```python
from build123d import *

# Parameters (mm, degrees)
BOSS_EXTRUDE1_DEPTH = 11.5
BOSS_EXTRUDE2_DEPTH = 22
SKETCH3_R           = 2.5
CUT_EXTRUDE1_DEPTH  = 4
SKETCH4_R           = 4.5
CUT_EXTRUDE2_DEPTH  = 5
SKETCH5_R           = 2.75
CUT_EXTRUDE3_DEPTH  = 125.343311555
SKETCH6_R           = 2.5
CUT_EXTRUDE4_DEPTH  = 79.78509189
CUT_EXTRUDE5_DEPTH  = 8.2
CUT_EXTRUDE6_DEPTH  = 9
FILLET1_R           = 5.05
FILLET2_R           = 5


with BuildPart() as part:
    # Sketch1 → Boss-Extrude1 (new body)
    with BuildSketch(Plane(origin=(0, 0, 0), x_dir=(1, 0, 0), z_dir=(0, 1, 0))):
        with BuildLine():
            Line((66.174969976, -35), (93.674969976, -35))
            ThreePointArc((93.674969976, -35), (98.07852804, 19.509032202), (73.150467337, 68.183642675))
            Line((73.150467337, 68.183642675), (47.743780193, 57.659848285))
            ThreePointArc((47.743780193, 57.659848285), (73.422287359, 14.604600997), (66.174969976, -35))
        make_face()
    extrude(amount=BOSS_EXTRUDE1_DEPTH)

    # Sketch2 → Boss-Extrude2 (add)
    with BuildSketch(Plane.XZ.offset(-11.5)):
        with BuildLine():
            Line((80.428539711, 23.5), (86.877787725, 23.5))
            ThreePointArc((86.877787725, 23.5), (85.091202872, 29.317012019), (82.915619759, 35))
            Line((82.915619759, 35), (76.428539711, 35))
            Line((76.428539711, 35), (76.428539711, 27.5))
            ThreePointArc((76.428539711, 27.5), (77.600112586, 24.671572875), (80.428539711, 23.5))
        make_face()
        with BuildLine():
            Line((60.086969148, -54.654623051), (57.216843406, -61.583719545))
            Line((57.216843406, -61.583719545), (63.210123888, -64.066217604))
            ThreePointArc((63.210123888, -64.066217604), (67.394885944, -59.648380938), (71.271549248, -54.957859017))
            Line((71.271549248, -54.957859017), (65.313221008, -52.489838651))
            ThreePointArc((65.313221008, -52.489838651), (62.251753549, -52.489838651), (60.086969148, -54.654623051))
        make_face()
    extrude(amount=-BOSS_EXTRUDE2_DEPTH)

    # Sketch3 → Cut-Extrude1 (cut)
    with BuildSketch(Plane(origin=(0, 33.5, 0), x_dir=(1, 0, 0), z_dir=(0, 1, 0))):
        with Locations(Location((63.782487278, 56.185356781, 0), (0, 0, 270))):
            Circle(SKETCH3_R)
        with Locations(Location((80.428539711, -27.5, 0), (0, 0, 270))):
            Circle(SKETCH3_R)
    extrude(amount=-CUT_EXTRUDE1_DEPTH, mode=Mode.SUBTRACT)

    # Sketch4 → Cut-Extrude2 (cut)
    with BuildSketch(Plane.XZ):
        with Locations(Location((91.060743988, 27, 0), (0, 0, 270))):
            Circle(SKETCH4_R)
        with Locations(Location((73.796704912, -59.792185441, 0), (0, 0, 270))):
            Circle(SKETCH4_R)
    extrude(amount=-CUT_EXTRUDE2_DEPTH, mode=Mode.SUBTRACT)

    # Sketch5 → Cut-Extrude3 (cut, through all)
    with BuildSketch(Plane.XZ.offset(-5)):
        with Locations(Location((91.060743988, 27, 0), (0, 0, 270))):
            Circle(SKETCH5_R)
        with Locations(Location((73.796704912, -59.792185441, 0), (0, 0, 270))):
            Circle(SKETCH5_R)
    extrude(amount=-CUT_EXTRUDE3_DEPTH, mode=Mode.SUBTRACT)

    # Sketch6 → Cut-Extrude4 (cut, through all)
    with BuildSketch(Plane(origin=(56.959375084, 0, -11.329924142), x_dir=(0.19509032201612866, 0, 0.9807852804032304), z_dir=(-0.9807852804032304, 0, 0.19509032201612866))):
        with Locations((0, 7.5)):
            Circle(SKETCH6_R)
    extrude(amount=-CUT_EXTRUDE4_DEPTH, mode=Mode.SUBTRACT)

    # Sketch8 → Cut-Extrude5 (cut)
    with BuildSketch(Plane(origin=(98.07852804, 0, -19.509032202), x_dir=(-0.19509032201612866, 0, -0.9807852804032304), z_dir=(0.9807852804032304, 0, -0.19509032201612866))):
        with BuildLine():
            Line((-4.5, 7.5), (-4.5, 11.5))
            Line((-4.5, 11.5), (4.5, 11.5))
            Line((4.5, 11.5), (4.5, 7.5))
            ThreePointArc((4.5, 7.5), (0, 3), (-4.5, 7.5))
        make_face()
    extrude(amount=-CUT_EXTRUDE5_DEPTH, mode=Mode.SUBTRACT)

    # Sketch7 → Cut-Extrude6 (cut)
    with BuildSketch(Plane(origin=(0, 11.5, 0), x_dir=(1, 0, 0), z_dir=(0, 1, 0))):
        Polygon((69.47485004, 18.968342244), (71.445262293, 9.062410912), (79.291544536, 10.623133488), (77.321132284, 20.52906482), align=None)
    extrude(amount=-CUT_EXTRUDE6_DEPTH, mode=Mode.SUBTRACT)

    # Fillet1
    # the kernel refuses this fillet: 5.05 mm, written as the material it adds along each edge
    with BuildSketch(Plane(origin=(61.857828731, 2.5, -7.155351805), x_dir=(0, 1, 0), z_dir=(0.9807852804032302, 0, -0.1950903220161298))) as fillet1_piece_1_section:
        with BuildLine():
            CenterArc((FILLET1_R, -FILLET1_R), FILLET1_R, 90, 90)
            Line((0, -FILLET1_R), (0, 0))
            Line((0, 0), (FILLET1_R, 0))
        make_face()
    fillet1_piece_1 = extrude(amount=30.40026249, mode=Mode.PRIVATE)
    fillet1_piece_1 = fillet1_piece_1 - Plane(origin=(0, 3.649852304, 0), x_dir=(0.6377681563457176, 0, -0.7702283938880625), z_dir=(0, -1, 0)) * Cylinder(74.860715007, 82, mode=Mode.PRIVATE)
    add(fillet1_piece_1)
    with BuildSketch(Plane(origin=(89.703546449, 2.5, -22.992080135), x_dir=(0, 1, 0), z_dir=(-0.9807852804032304, 0, 0.19509032201612841))) as fillet1_piece_2_section:
        with BuildLine():
            CenterArc((FILLET1_R, -FILLET1_R), FILLET1_R, 90, 90)
            Line((0, -FILLET1_R), (0, 0))
            Line((0, 0), (FILLET1_R, 0))
        make_face()
    fillet1_piece_2 = extrude(amount=30.40026249, mode=Mode.PRIVATE)
    fillet1_piece_2 = fillet1_piece_2 - Plane(origin=(0, 3.643295327, 0), x_dir=(0.6377681563457176, 0, -0.7702283938880625), z_dir=(0, -1, 0)) * Cylinder(74.860715007, 82, mode=Mode.PRIVATE)
    add(fillet1_piece_2)

    # Fillet2
    fillet2_edges = [part.edges().sort_by_distance(p)[0] for p in [
        (66.174969976, 5.75, 35),
        (47.743780193, 5.75, -57.659848285),
    ]]
    fillet(fillet2_edges, radius=FILLET2_R)


solid = part.part
```
Could you check a few things on this model? Use its own coordinates, in mm. A direction names the side the tool comes from. Coordinates: 2 decimals unless noted, no trailing zeros. Loops run counter-clockwise (first coordinate to the right, second up) from the corner with the lowest first, then second, coordinate; pieces in that order, holes last.
1) Will these pins go through, and if not, where does the flat tip stop? pin 1 Ø4 at (x, z) = (80.43, 27.5) entering from +Y; pin 2 Ø2 at (y, z) = (11.5, -33.5) entering from -X; pin 3 Ø4.5 at (x, z) = (91.06, 27) entering from +Y; pin 4 Ø4 at (y, z) = (12, 10) entering from -X.
Reported:
pin 1: stops at y = 29.5
pin 2: stops at x = 66.44
pin 3: passes through
pin 4: stops at x = 73.9
2) Imagine slicing it at B-B (y = 31). List the corners of the cut face in (x, z) for me, and give its area (3 significant figures).
Reported:
outline: (57.22, -61.58) - (63.21, -64.07) arc R90 ccw to (71.27, -54.96) - (65.31, -52.49) arc R4 ccw to (60.09, -54.65) - close; (76.43, 27.5) arc R4 ccw to (80.43, 23.5) - (86.88, 23.5) arc R90 ccw to (82.92, 35) - (76.43, 35) - close; hole circle Ø5 at (63.78, -56.19); hole circle Ø5 at (80.43, 27.5)
area: 152 mm2
3) Thinking about a two-plate mould opening in Z: for faces 1 (the face through (69.83, 5.83, 32.74)), 2 (the face through (77.57, 22.35, 24.7)), 3 (the face through (85.119, 22.346, 29.236)), which applies, released by +Z, released by -Z, zero draft, split by the parting line, or undercut?
Reported:
face 1: undercut
face 2: released by -Z
face 3: released by +Z
4) Imagine slicing it at C-C (z = 2). List the corners of the cut face in (x, y) for me, and give its area (3 significant figures).
Reported:
outline: (74.83, 0) - (99.98, 0) - (99.98, 11.5) - (74.83, 11.5) - close
area: 289 mm2
5) Which directions (+Z, -Z, +X, -X, +Y, -Y) give clear straight access to the entire face, cutting with the end or side of a thin tool? Please do faces 4 (the face through (76, 5, -62)), 5 (the face through (80, 29.5, 27)), 6 (the face through (84, 22, 23.5)), 7 (the face through (68.33, 22.35, -53.74)).
Reported:
face 4: -Y
face 5: +Y
face 6: -Z, +X, -X, +Y
face 7: +Z, +X, +Y
6) Imagine slicing it at D-D (z = -50). List the corners of the cut face in (x, y) for me.
Reported:
outline: (55.71, 0) - (86.6, 0) - (86.6, 11.5) - (55.71, 11.5) - close
7) Please list where these lines run through material, in increasing order: line 1 along X through (y, z) = (2.7, 27); line 2 along Y through (x, z) = (88, -18.5); line 3 along Y through (x, z) = (89.5, -14).
Reported:
line 1: x = 69.82 to 86.56, 95.56 to 96.29
line 2: y = 0 to 5.2, 9.8 to 11.5
line 3: y = 0 to 11.5
8) Imagine slicing it at A-A (y = 24.5). List the corners of the cut face in (x, z) for me.
Reported:
outline: (57.22, -61.58) - (63.21, -64.07) arc R90 ccw to (71.27, -54.96) - (65.31, -52.49) arc R4 ccw to (60.09, -54.65) - close; (76.43, 27.5) arc R4 ccw to (80.43, 23.5) - (86.88, 23.5) arc R90 ccw to (82.92, 35) - (76.43, 35) - close
